from build123d import *

# Parameters (mm, degrees)
ESBO_O23_W                     = 44.3
ESBO_O23_H                     = 11.5
ESBO_O23_R                     = 2
FLANGE_BASE2_DEPTH             = 3
ARESTA_FLANGE1_STRIP_W         = 13.4732
ARESTA_FLANGE1_STRIP_H         = 3
ARESTA_FLANGE1_STRIP_CUT_DEPTH = 44.3
ARESTA_FLANGE1_DEPTH           = 44.3
CORTE_EXTRUS_O1_REACH          = 41.939
CORTE_EXTRUS_O2_REACH          = 41.939
ESBO_O33_R                     = 1.5
ESBO_O33_W                     = 10
ESBO_O33_H                     = 11.0034
FILETE1_START                  = -5
FILETE1_DEPTH                  = 12.011168151
FILETE1_START_2                = 4.011168151
FILETE1_2_DEPTH                = 3
FILETE1_3_DEPTH                = 3
FILETE1_START_3                = -4
FILETE1_4_DEPTH                = 4.7366001
ESBO_O34_W                     = 24.3
ESBO_O34_H                     = 4.7634
CORTE_EXTRUS_O3_DEPTH          = 39.884804768
FILETE2_R                      = 2


with BuildPart() as part:
    # Flange-base2: sheet metal written as solids
    # Esboço23 → Flange-base2 (new body)
    with BuildSketch(Plane(origin=(0, 0, 0), x_dir=(1, 0, 0), z_dir=(0, 1, 0))):
        with Locations((13.143114832, -1.261168151)):
            Rectangle(ESBO_O23_W, ESBO_O23_H)
        with Locations(Location((-4.006885168, 0.488831849, 0), (0, 0, 270))):
            Circle(ESBO_O23_R, mode=Mode.SUBTRACT)
        with Locations(Location((30.293114832, 0.488831849, 0), (0, 0, 90))):
            Circle(ESBO_O23_R, mode=Mode.SUBTRACT)
    extrude(amount=-FLANGE_BASE2_DEPTH)

    # Aresta-Flange1: sheet metal written as solids
    # Aresta-Flange1 strip (on a plane across the edge) → Aresta-Flange1 strip cut (cut)
    with BuildSketch(Plane(origin=(-9.006885168, 0, 7.011168151), x_dir=(0, 0, -1), z_dir=(1, 0, 0))):
        with Locations((-3, -1.5)):
            Rectangle(ARESTA_FLANGE1_STRIP_W, ARESTA_FLANGE1_STRIP_H)
    extrude(amount=ARESTA_FLANGE1_STRIP_CUT_DEPTH, mode=Mode.SUBTRACT)

    # Aresta-Flange1 section (on a plane across the edge) → Aresta-Flange1 (add)
    with BuildSketch(Plane(origin=(-9.006885168, 0, 7.011168151), x_dir=(0, 0, -1), z_dir=(1, 0, 0))):
        with BuildLine():
            Line((0, 0.7366), (0, 14.74))
            Line((0, 14.74), (3, 14.74))
            Line((3, 14.74), (3, 0.7366))
            ThreePointArc((3, 0.7366), (3.215745145, 0.215745145), (3.7366, 0))
            Line((3.7366, 0), (3.7366, -3))
            ThreePointArc((3.7366, -3), (1.094424801, -1.905575199), (0, 0.7366))
        make_face()
    extrude(amount=ARESTA_FLANGE1_DEPTH)

    # Esboço31 → Corte-extrusão1 (cut, up to next)
    with BuildSketch(Plane.XY.offset(7.011168151), mode=Mode.PRIVATE) as corte_extrus_o1_sk1:
        with BuildLine():
            Line((5.143114832, 14.74), (5.143114832, 11.99))
            Line((5.143114832, 11.99), (3.393114832, 11.99))
            ThreePointArc((3.393114832, 11.99), (0.641414832, 9.2383), (3.393114832, 6.4866))
            Line((3.393114832, 6.4866), (5.143114832, 6.4866))
            Line((5.143114832, 6.4866), (5.143114832, 0.7366))
            Line((5.143114832, 0.7366), (-9.006885168, 0.7366))
            Line((-9.006885168, 0.7366), (-9.006885168, 14.74))
            Line((-9.006885168, 14.74), (5.143114832, 14.74))
        make_face()
    corte_extrus_o1_tool1 = extrude(corte_extrus_o1_sk1.sketch, amount=-CORTE_EXTRUS_O1_REACH, mode=Mode.PRIVATE) & part.part
    # Esboço31 → Corte-extrusão1 (cut, up to next)
    with BuildSketch(Plane.XY.offset(7.011168151), mode=Mode.PRIVATE) as corte_extrus_o1_sk2:
        with BuildLine():
            Line((21.143114832, 6.4866), (21.143114832, 0.7366))
            Line((21.143114832, 0.7366), (35.293114832, 0.7366))
            Line((35.293114832, 0.7366), (35.293114832, 14.74))
            Line((35.293114832, 14.74), (21.143114832, 14.74))
            Line((21.143114832, 14.74), (21.143114832, 11.99))
            Line((21.143114832, 11.99), (22.893114832, 11.99))
            ThreePointArc((22.893114832, 11.99), (25.644814832, 9.2383), (22.893114832, 6.4866))
            Line((22.893114832, 6.4866), (21.143114832, 6.4866))
        make_face()
    corte_extrus_o1_tool2 = extrude(corte_extrus_o1_sk2.sketch, amount=-CORTE_EXTRUS_O1_REACH, mode=Mode.PRIVATE) & part.part
    add(corte_extrus_o1_tool1.solids().sort_by_distance((-2.549902, 7.555498, 7.011168))[0], mode=Mode.SUBTRACT)
    add(corte_extrus_o1_tool2.solids().sort_by_distance((28.836132, 7.555498, 7.011168))[0], mode=Mode.SUBTRACT)

    # Esboço33 → Corte-extrusão2 (cut, up to next)
    with BuildSketch(Plane.XY.offset(7.011168151), mode=Mode.PRIVATE) as corte_extrus_o2_sk1:
        with Locations((3.393114832, 9.2383)):
            Circle(ESBO_O33_R)
    corte_extrus_o2_tool1 = extrude(corte_extrus_o2_sk1.sketch, amount=-CORTE_EXTRUS_O2_REACH, mode=Mode.PRIVATE) & part.part
    # Esboço33 → Corte-extrusão2 (cut, up to next)
    with BuildSketch(Plane.XY.offset(7.011168151), mode=Mode.PRIVATE) as corte_extrus_o2_sk2:
        with Locations(Location((22.893114832, 9.2383, 0), (0, 0, 180))):
            Circle(ESBO_O33_R)
    corte_extrus_o2_tool2 = extrude(corte_extrus_o2_sk2.sketch, amount=-CORTE_EXTRUS_O2_REACH, mode=Mode.PRIVATE) & part.part
    # Esboço33 → Corte-extrusão2 (cut, up to next)
    with BuildSketch(Plane.XY.offset(7.011168151), mode=Mode.PRIVATE) as corte_extrus_o2_sk3:
        with Locations((13.143114832, 9.2383)):
            Rectangle(ESBO_O33_W, ESBO_O33_H)
    corte_extrus_o2_tool3 = extrude(corte_extrus_o2_sk3.sketch, amount=-CORTE_EXTRUS_O2_REACH, mode=Mode.PRIVATE) & part.part
    add(corte_extrus_o2_tool1.solids().sort_by_distance((3.393115, 9.2383, 7.011168))[0], mode=Mode.SUBTRACT)
    add(corte_extrus_o2_tool2.solids().sort_by_distance((22.893115, 9.2383, 7.011168))[0], mode=Mode.SUBTRACT)
    add(corte_extrus_o2_tool3.solids().sort_by_distance((13.143115, 9.2383, 7.011168))[0], mode=Mode.SUBTRACT)

    # Filete1: read off the stored shape, not the designer's step
    # Filete1 outline → Filete1 (cut)
    with BuildSketch(Plane.XY.offset(FILETE1_START)):
        with BuildLine():
            Line((-9.006885168, 0.7366), (-9.006885168, -1.2634))
            ThreePointArc((-9.006885168, -1.2634), (-8.42109873, 0.150813562), (-7.006885168, 0.7366))
            Line((-7.006885168, 0.7366), (-9.006885168, 0.7366))
        make_face()
        with BuildLine():
            ThreePointArc((33.293114832, 0.7366), (34.707328395, 0.150813562), (35.293114832, -1.2634))
            Line((35.293114832, -1.2634), (35.293114832, 0.7366))
            Line((35.293114832, 0.7366), (33.293114832, 0.7366))
        make_face()
    extrude(amount=FILETE1_DEPTH, mode=Mode.SUBTRACT)

    # Filete1 2 outline → Filete1 2 (add)
    with BuildSketch(Plane.XY.offset(FILETE1_START_2)):
        with BuildLine():
            ThreePointArc((5.143114832, 2.7366), (4.557328394, 1.322386438), (3.143114832, 0.7366))
            Line((3.143114832, 0.7366), (5.143114832, 0.7366))
            Line((5.143114832, 0.7366), (5.143114832, 2.7366))
        make_face()
        with BuildLine():
            Line((21.143114832, 0.7366), (23.143114832, 0.7366))
            ThreePointArc((23.143114832, 0.7366), (21.72890127, 1.322386438), (21.143114832, 2.7366))
            Line((21.143114832, 2.7366), (21.143114832, 0.7366))
        make_face()
        with BuildLine():
            Line((8.143114832, 3.7366), (10.143114832, 3.7366))
            ThreePointArc((10.143114832, 3.7366), (8.72890127, 4.322386438), (8.143114832, 5.7366))
            Line((8.143114832, 5.7366), (8.143114832, 3.7366))
        make_face()
        with BuildLine():
            ThreePointArc((18.143114832, 5.7366), (17.557328394, 4.322386437), (16.143114832, 3.7366))
            Line((16.143114832, 3.7366), (18.143114832, 3.7366))
            Line((18.143114832, 3.7366), (18.143114832, 5.7366))
        make_face()
    extrude(amount=FILETE1_2_DEPTH)

    # Filete1 3 outline → Filete1 3 (add)
    with BuildSketch(Plane.XY.offset(FILETE1_START_2)):
        with BuildLine():
            ThreePointArc((22.893114832, 11.99), (22.96552716, 11.989047052), (23.037889334, 11.986188868))
            ThreePointArc((23.037889334, 11.986188868), (21.69217531, 12.606910766), (21.143114832, 13.983418849))
            Line((21.143114832, 13.983418849), (21.143114832, 11.99))
            Line((21.143114832, 11.99), (22.893114832, 11.99))
        make_face()
        with BuildLine():
            ThreePointArc((21.143114832, 4.493181151), (21.69217531, 5.869689234), (23.037889334, 6.490411131))
            ThreePointArc((23.037889334, 6.490411131), (22.96552716, 6.487552948), (22.893114832, 6.4866))
            Line((22.893114832, 6.4866), (21.143114832, 6.4866))
            Line((21.143114832, 6.4866), (21.143114832, 4.493181151))
        make_face()
        with BuildLine():
            ThreePointArc((5.143114832, 13.983418849), (4.594054355, 12.606910766), (3.248340331, 11.986188869))
            ThreePointArc((3.248340331, 11.986188869), (3.320702504, 11.989047052), (3.393114832, 11.99))
            Line((3.393114832, 11.99), (5.143114832, 11.99))
            Line((5.143114832, 11.99), (5.143114832, 13.983418849))
        make_face()
        with BuildLine():
            ThreePointArc((3.248340331, 6.490411131), (4.594054355, 5.869689234), (5.143114832, 4.493181151))
            Line((5.143114832, 4.493181151), (5.143114832, 6.4866))
            Line((5.143114832, 6.4866), (3.393114832, 6.4866))
            ThreePointArc((3.393114832, 6.4866), (3.320702504, 6.487552948), (3.248340331, 6.490411131))
        make_face()
    extrude(amount=FILETE1_3_DEPTH)

    # Filete1 4 outline → Filete1 4 (cut)
    with BuildSketch(Plane(origin=(0, 0, 0), x_dir=(1, 0, 0), z_dir=(0, 1, 0)).offset(FILETE1_START_3)):
        with BuildLine():
            Line((35.293114832, 4.488831849), (33.293114832, 4.488831849))
            ThreePointArc((33.293114832, 4.488831849), (34.707328395, 3.903045412), (35.293114832, 2.488831849))
            Line((35.293114832, 2.488831849), (35.293114832, 4.488831849))
        make_face()
        with BuildLine():
            ThreePointArc((-9.006885168, 2.488831849), (-8.421098731, 3.903045412), (-7.006885168, 4.488831849))
            Line((-7.006885168, 4.488831849), (-9.006885168, 4.488831849))
            Line((-9.006885168, 4.488831849), (-9.006885168, 2.488831849))
        make_face()
    extrude(amount=FILETE1_4_DEPTH, mode=Mode.SUBTRACT)

    # Esboço34 → Corte-extrusão3 (cut, through all)
    with BuildSketch(Plane(origin=(0, 0, 0), x_dir=(1, 0, 0), z_dir=(0, 1, 0))):
        with Locations((13.143114832, 2.107131849)):
            Rectangle(ESBO_O34_W, ESBO_O34_H)
    extrude(amount=-CORTE_EXTRUS_O3_DEPTH, mode=Mode.SUBTRACT)

    # Filete2
    # the kernel refuses this fillet: 2 mm, written as the material it adds along each edge
    with BuildSketch(Plane(origin=(0.993114832, 0, 0.274568151), x_dir=(0, 0, -1), z_dir=(0, -1, 0))) as filete2_piece_1:
        with BuildLine():
            CenterArc((FILETE2_R, FILETE2_R), FILETE2_R, 180, 90)
            Line((0, FILETE2_R), (0, 0))
            Line((0, 0), (FILETE2_R, 0))
        make_face()
    extrude(amount=3)
    with BuildSketch(Plane(origin=(25.293114832, 0, 0.274568151), x_dir=(0, 0, -1), z_dir=(0, -1, 0))) as filete2_piece_2:
        with BuildLine():
            CenterArc((FILETE2_R, -FILETE2_R), FILETE2_R, 90, 90)
            Line((0, -FILETE2_R), (0, 0))
            Line((0, 0), (FILETE2_R, 0))
        make_face()
    extrude(amount=3)
    # the kernel refuses this fillet: 2 mm, written as the material it takes off along each edge
    with BuildSketch(Plane(origin=(5.143114832, 14.74, 11.515742565), x_dir=(1, 0, 0), z_dir=(0, 0, -1))) as filete2_2_piece_1:
        with BuildLine():
            CenterArc((1.801829766, 2), FILETE2_R, 198.110746947, 71.889253053)
            Line((-0.099085117, 1.378290576), (-0.289176606, 1.316119634))
            ThreePointArc((-0.289176606, 1.316119634), (-0.2, 0.756581151), (-0.2, 0))
            Line((-0.2, 0), (0, -0.2))
            Line((0, -0.2), (1.801829766, -0.2))
            Line((1.801829766, -0.2), (1.801829766, 0))
        make_face()
    extrude(amount=12.009148828, mode=Mode.SUBTRACT)
    with BuildSketch(Plane(origin=(21.143114832, 14.74, 11.515742565), x_dir=(0.07170480855584176, -0.9974258972124044, 0), z_dir=(0, 0, -1))) as filete2_2_piece_2:
        with BuildLine():
            CenterArc((1.865651936, 1.940601288), FILETE2_R, 184.111911668, 71.889253032)
            Line((-0.129199858, 1.797191671), (-0.328685038, 1.782850709))
            Line((-0.328685038, 1.782850709), (-0.199485179, -0.014340962))
            Line((-0.199485179, -0.014340962), (0.014340962, -0.199485179))
            ThreePointArc((0.014340962, -0.199485179), (0.768974595, -0.145234673), (1.333467159, -0.194060129))
            Line((1.333467159, -0.194060129), (1.381847593, 0))
        make_face()
    extrude(amount=12.009148828, mode=Mode.SUBTRACT)
    with BuildSketch(Plane(origin=(8.143114832, 14.74, 12.011168151), x_dir=(0, -1, 0), z_dir=(0, 0, -1)), Plane(origin=(18.143114832, 14.74, 12.011168151), x_dir=(1, 0, 0), z_dir=(0, 0, -1)), Plane(origin=(25.293114832, 5, -4.488831849), x_dir=(1, 0, 0), z_dir=(0, -1, 0))) as filete2_2_piece_3:
        with BuildLine():
            CenterArc((FILETE2_R, FILETE2_R), FILETE2_R, 180, 90)
            Line((0, FILETE2_R), (0, 0))
            Line((0, 0), (FILETE2_R, 0))
        make_face()
    extrude(amount=13, mode=Mode.SUBTRACT)
    with BuildSketch(Plane(origin=(0.993114832, 5, -4.488831849), x_dir=(-1, 0, 0), z_dir=(0, -1, 0))) as filete2_2_piece_4:
        with BuildLine():
            CenterArc((FILETE2_R, -FILETE2_R), FILETE2_R, 90, 90)
            Line((0, -FILETE2_R), (0, 0))
            Line((0, 0), (FILETE2_R, 0))
        make_face()
    extrude(amount=13, mode=Mode.SUBTRACT)


solid = part.part
Model file for the job. Use its own axes, mm. A direction names the side the tool comes from. Coordinates: 2 decimals unless noted, no trailing zeros. Write each loop counter-clockwise with the first axis right and the second up, starting at its lowest first coordinate (ties: lowest second). Pieces come first, ordered by that corner, then holes. Notation, with made-up numbers: (-2.75, 39) -> (55.25, 39) arc R21 cw to (55.25, 64) -> close; hole circle Ø4 at (48.5, 21.25). An arc over 180 degrees is marked (long way). One line per item, written item: value. Start each with the question number.
1) Slice it at D-D on x = -3. Write the cut outline in (y, z).
2) Which spindle directions (+Z, -Z, +X, -X, +Y, -Y) get a long thin tool onto all of the face, cutting with end or side? Do faces 1 (the face through (0.39, -1.48, -3.92)), 2 (the face through (13, 3, 4.011)), 3 (the face through (4.573, 1.338, 5.49)), 4 (the face through (8.74, 4.31, 5.49)). Say none if no direction does.
3) Probe probe 1 along Y at (x, z) = (-6, 1); probe 2 along Z at (x, y) = (30.5, -1); probe 3 along Z at (x, y) = (20, 3). List the from-to ranges inside material, lowest first.
4) Pull direction Y, two halves, no side cores. Call faces 5 (the face through (17.573, 4.338, 5.49)), 6 (the face through (8.143, 9, 6)), 7 (the face through (21.143, 4, 6)): +Y half, -Y half, draft (parallel to the pull), parting line (faces both ways), or undercut.
5) Flat gauge pins, fed straight in: pin 1 Ø1.5 at (y, z) = (8.5, 6) entering from -X; pin 2 Ø1.5 at (x, z) = (-1, 5) entering from +Y; pin 3 Ø7 at (x, y) = (15, 9.5) entering from -Z; pin 4 Ø2.5 at (x, z) = (-4.01, -0.49) entering from -Y. Where does each tip first touch, or does it go through?
6) Slice it at C-C on z = 5.25. Write the cut outline in (x, y).
7) Slice it at A-A on x = 13.5. Write the cut outline in (y, z), then the cut area to 3 significant figures.
8) Slice it at B-B on z = -3.25. Write the cut outline in (x, y).
Answers follow:
1. outline: (-3, -4.49) -> (0, -4.49) -> (0, -2.22) -> (-3, -2.22) -> close; (-3, 1.24) -> (0, 1.24) -> (0, 3.27) arc R0.74 cw to (0.74, 4.01) -> (0.74, 7.01) arc R3.74 ccw to (-3, 3.27) -> close
2. face 1: -Z, +Y, -Y
2. face 2: -Z, +X, -X, +Y
2. face 3: +Z, -Z, -X
2. face 4: +Z, -Z, +Y
3. probe 1: -3 to 0
3. probe 2: -4.49 to -2.48, 1.5 to 6.58
3. probe 3: 4.01 to 7.01
4. face 5: +Y half
4. face 6: draft
4. face 7: undercut
5. pin 1: x = 0.64
5. pin 2: y = 0.74
5. pin 3: z = 4.01
5. pin 4: through
6. outline: (-9.01, -2.44) -> (35.29, -2.44) -> (35.29, -1.26) arc R2 ccw to (33.29, 0.74) -> (23.14, 0.74) arc R2 cw to (21.14, 2.74) -> (21.14, 4.49) arc R2 cw to (23.04, 6.49) arc R2.75 ccw to (23.04, 11.99) arc R2 cw to (21.24, 13.36) arc R2 ccw to (19.74, 14.7) arc R2 ccw to (18.14, 12.74) -> (18.14, 5.74) arc R2 cw to (16.14, 3.74) -> (10.14, 3.74) arc R2 cw to (8.14, 5.74) -> (8.14, 12.74) arc R2 ccw to (6.54, 14.7) arc R2 ccw to (5.04, 13.36) arc R2 cw to (3.25, 11.99) arc R2.75 ccw to (3.25, 6.49) arc R2 cw to (5.14, 4.49) -> (5.14, 2.74) arc R2 cw to (3.14, 0.74) -> (-7.01, 0.74) arc R2 ccw to (-9.01, -1.26) -> close; hole circle Ø3 at (3.39, 9.24); hole circle Ø3 at (22.89, 9.24)
7. outline: (-3, 0.27) -> (0, 0.27) -> (0, 3.27) arc R0.74 cw to (0.74, 4.01) -> (3.74, 4.01) -> (3.74, 7.01) -> (0.74, 7.01) arc R3.74 ccw to (-3, 3.27) -> close
7. area: 28.5 mm2
8. outline: (-8.86, -3) -> (0.84, -3) -> (0.84, 0) -> (-8.56, 0) arc R2 ccw to (-8.86, -0.5) -> close; (25.44, -3) -> (35.14, -3) -> (35.14, -0.5) arc R2 ccw to (34.84, 0) -> (25.44, 0) -> close
